from build123d import *

# Parameters (mm, degrees)
SKETCH1_R                 = 30.95625
BOSS_EXTRUDE1_DEPTH       = 50.8
CUT_EXTRUDE1_DEPTH        = 3.9624
CUT_EXTRUDE2_DEPTH        = 86.860858779
SKETCH4_R                 = 19.05
CUT_EXTRUDE3_DEPTH        = 60.630735383
SKETCH6_R                 = 23.8125
CUT_EXTRUDE4_DEPTH        = 44.45
F_4_40_TAPPED_HOLE1_D     = 2.2606
F_4_40_TAPPED_HOLE1_DEPTH = 7.62
F_4_40_TAPPED_HOLE1_TIP   = 0.679152758
SKETCH10_R                = 40.48125
BOSS_EXTRUDE3_DEPTH       = 4.7625
FILLET1_R                 = 5.08
CIRPATTERN1_COUNT         = 2
CIRPATTERN1_ANGLE         = 60
SKETCH15_R                = 3.9624
CUT_EXTRUDE5_DEPTH        = 5.08


with BuildPart() as part:
    # Sketch1 → Boss-Extrude1 (new body)
    with BuildSketch(Plane.XY):
        Circle(SKETCH1_R)
    extrude(amount=BOSS_EXTRUDE1_DEPTH)

    # Sketch2 → Cut-Extrude1 (cut)
    with BuildSketch(Plane(origin=(0, 0, 0), x_dir=(-1, 0, 0), z_dir=(0, 0, -1))):
        with BuildLine():
            Line((-18.3261, -22.2885), (18.3261, -22.2885))
            ThreePointArc((18.3261, -22.2885), (21.12793991, -21.12793991), (22.2885, -18.3261))
            Line((22.2885, -18.3261), (22.2885, 18.3261))
            ThreePointArc((22.2885, 18.3261), (21.12793991, 21.12793991), (18.3261, 22.2885))
            Line((18.3261, 22.2885), (-18.3261, 22.2885))
            ThreePointArc((-18.3261, 22.2885), (-21.12793991, 21.12793991), (-22.2885, 18.3261))
            Line((-22.2885, 18.3261), (-22.2885, -18.3261))
            ThreePointArc((-22.2885, -18.3261), (-21.12793991, -21.12793991), (-18.3261, -22.2885))
        make_face()
    extrude(amount=-CUT_EXTRUDE1_DEPTH, mode=Mode.SUBTRACT)

    # Sketch3 → Cut-Extrude2 (cut, through all)
    with BuildSketch(Plane(origin=(30.95625, 0, 0), x_dir=(0, 0, -1), z_dir=(1, 0, 0))):
        with BuildLine():
            Line((-44.45, 25.4), (0, 30.95625))
            Line((0, 30.95625), (-50.8, 30.95625))
            Line((-50.8, 30.95625), (-50.8, -30.95625))
            Line((-50.8, -30.95625), (0, -30.95625))
            Line((0, -30.95625), (-44.45, -25.4))
            ThreePointArc((-44.45, -25.4), (-19.05, 0), (-44.45, 25.4))
        make_face()
    extrude(amount=-CUT_EXTRUDE2_DEPTH, mode=Mode.SUBTRACT)

    # Sketch4 → Cut-Extrude3 (cut, through all)
    with BuildSketch(Plane(origin=(0, 0, 3.9624), x_dir=(-1, 0, 0), z_dir=(0, 0, -1))):
        Circle(SKETCH4_R)
    extrude(amount=-CUT_EXTRUDE3_DEPTH, mode=Mode.SUBTRACT)

    # Sketch6 → Cut-Extrude4 (cut)
    with BuildSketch(Plane.XY.offset(50.8)):
        Circle(SKETCH6_R)
    extrude(amount=-CUT_EXTRUDE4_DEPTH, mode=Mode.SUBTRACT)

    # #4-40 Tapped Hole1
    with Locations(Plane(origin=(0, 0, 3.9624), x_dir=(-1, 0, 0), z_dir=(0, 0, -1))):
        with Locations((-18.2626, 18.2626), (18.2626, 18.2626), (18.2626, -18.2626), (-18.2626, -18.2626)):
            Hole(F_4_40_TAPPED_HOLE1_D / 2, depth=F_4_40_TAPPED_HOLE1_DEPTH)
            with Locations((0, 0, -(F_4_40_TAPPED_HOLE1_DEPTH + F_4_40_TAPPED_HOLE1_TIP / 2))):  # 118° drill point
                Cone(0, F_4_40_TAPPED_HOLE1_D / 2, F_4_40_TAPPED_HOLE1_TIP, mode=Mode.SUBTRACT)

    # Sketch10 → Boss-Extrude3 (add)
    with BuildSketch(Plane(origin=(0, 0, 0), x_dir=(-1, 0, 0), z_dir=(0, 0, -1))):
        Circle(SKETCH10_R)
        with BuildLine():
            Line((-17.695463093, 25.4), (17.695463093, 25.4))
            ThreePointArc((17.695463093, 25.4), (30.95625, 0), (17.695463093, -25.4))
            Line((17.695463093, -25.4), (-17.695463093, -25.4))
            ThreePointArc((-17.695463093, -25.4), (-30.95625, 0), (-17.695463093, 25.4))
        make_face(mode=Mode.SUBTRACT)
    extrude(amount=-BOSS_EXTRUDE3_DEPTH)

    # Fillet1
    fillet1_edges = [part.edges().sort_by_distance(p)[0] for p in [
        (30.95625, 0, 4.7625),
        (-30.95625, 0, 4.7625),
        (0, -30.3609375, 4.7625),
        (0, 30.3609375, 4.7625),
    ]]
    fillet(fillet1_edges, radius=FILLET1_R)

    # Sketch13 → #8 Clearance Hole1 (revolve, cut)
    with BuildSketch(Plane(origin=(-18.415, 31.895715621, 4.7625), x_dir=(0, -1, 0), z_dir=(1, 0, 0))):
        Polygon((0, 0), (0, 26.750674586), (2.2479, 25.4), (2.2479, 0), align=None)
    f_8_clearance_hole1 = revolve(axis=Axis((-18.415, 31.895715621, 11.1125), (0, 0, -1)), mode=Mode.SUBTRACT)

    # CirPattern1: #8 Clearance Hole1 ×2 about axis
    cirpattern1_axis = Axis((0, 0, 4.7625), (0, 0, -1))
    for i in range(1, CIRPATTERN1_COUNT):
        add(f_8_clearance_hole1.rotate(cirpattern1_axis, i * CIRPATTERN1_ANGLE / (CIRPATTERN1_COUNT - 1)), mode=Mode.SUBTRACT)

    # Mirror1: #8 Clearance Hole1 across plane
    add(f_8_clearance_hole1.mirror(Plane.ZX), mode=Mode.SUBTRACT)

    # Mirror1 copy 1 sketch → Mirror1 copy 1 (revolve, cut)
    with BuildSketch(Plane(origin=(18.415, -31.895715621, 4.7625), x_dir=(-0.8660254037844399, 0.4999999999999978, 0), z_dir=(0.4999999999999978, 0.8660254037844399, 0))):
        Polygon((0, 0), (0, -26.750674586), (2.2479, -25.4), (2.2479, 0), align=None)
    revolve(axis=Axis((18.415, -31.895715621, 11.1125), (0, 0, 1)), mode=Mode.SUBTRACT)

    # Sketch15 → Cut-Extrude5 (cut)
    with BuildSketch(Plane.XY.offset(9.8425)):
        with Locations((-18.415, 31.895715621)):
            Circle(SKETCH15_R)
        with Locations((18.415, 31.895715621)):
            Circle(SKETCH15_R)
        with Locations((18.415, -31.895715621)):
            Circle(SKETCH15_R)
        with Locations((-18.415, -31.895715621)):
            Circle(SKETCH15_R)
    extrude(amount=-CUT_EXTRUDE5_DEPTH, mode=Mode.SUBTRACT)


solid = part.part
Geometry: final body of the model. Coordinates: model frame, mm. A direction names the side the tool comes from. Give positions to 0.01 mm unless a question says otherwise; leave off trailing zeros. Write each loop counter-clockwise with the first axis right and the second up, starting at its lowest first coordinate (ties: lowest second). Pieces come first, ordered by that corner, then holes. Notation, with made-up numbers: (86.25, 8) - (141.25, 8) arc R10 cw to (141.25, 23) - close; hole circle Ø1 at (19, 37). An arc over 180 degrees is marked (long way). Return JSON: item names as keys, results as strings. Group by question number.
1) Section A-A on x = 0. Return the cut outline in (y, z), plus the area to 3 significant figures.
2) Section D-D on z = 15.5. Return the cut outline in (x, y) (1 decimal), plus the area to 3 significant figures.
3) Section B-B on y = 0. Return the cut outline in (x, z).
4) Set-up query: faces 1 (the cylindrical face through (30.95, -0.56, 15.37)), 2 (the cylindrical face through (-17.741, -19.265, 7.826)), 3 (the cylindrical face through (-17.551, 16.094, 17.934)), 4 (the cylindrical face through (15.12, -11.59, 5.14)). Return all of +Z, -Z, +X, -X, +Y, -Y with unobstructed straight access to the full face (end or side cutting, diameter ignored); none if empty.
5) Mould query, pull axis Y, two halves, no side actions, for faces 5 (the cylindrical face through (18.784, -19.265, 7.826)), 6 (the flat face through (-26, 1, 0)), 7 (the cylindrical face through (-30.95, 0.56, 15.37)), 8 (the cylindrical face through (-13.614, -20.485, 29.432)). Classes: released by +Y, released by -Y, zero draft, split by the parting line, or undercut.
6) First-contact query: P1, Ø2.5, axis at x = 18.26, y = -18.26, coming from the -Z side; P2, Ø8, axis at x = 10.5, z = 8, coming from the +Y side; P3, Ø14.5, axis at x = -11, y = 11, coming from the +Z side; P4, Ø5, axis at x = 18.41, y = 31.9, coming from the -Z side. Flat tips, straight axial feed; report the tip coordinate or a pass-through.
7) Section C-C on z = 33.5. Return the cut outline in (x, y) (1 decimal), plus the area to 3 significant figures.
8) Line query: line 1 (Y direction, x = 3, z = 12); line 2 (Y direction, x = -17, z = 6.5); line 3 (Z direction, x = 20, y = 0). Output: solid intervals per line, ascending.
Filled in:
{
 "1": {"outline": "(-40.48, 0) - (-22.29, 0) - (-22.29, 3.96) - (-19.05, 3.96) - (-19.05, 6.35) - (-23.81, 6.35) - (-23.81, 35.61) arc R25.4 cw to (-25.4, 44.45) - (-29.8, 9.21) arc R5.08 cw to (-34.85, 4.76) - (-40.48, 4.76) - close; (19.05, 3.96) - (22.29, 3.96) - (22.29, 0) - (40.48, 0) - (40.48, 4.76) - (34.85, 4.76) arc R5.08 cw to (29.8, 9.21) - (25.4, 44.45) arc R25.4 cw to (23.81, 35.61) - (23.81, 6.35) - (19.05, 6.35) - close", "area": "506 mm^2"},
 "2": {"outline": "(-10.8, -29) - (10.8, -29) arc R31 ccw to (10.8, 29) - (-10.8, 29) arc R31 ccw to start; hole circle Ø47.6 at (0, 0)", "area": "1,170 mm^2"},
 "3": {"outline": "(-40.48, 0) - (-22.29, 0) - (-22.29, 3.96) - (-19.05, 3.96) - (-19.05, 6.35) - (-23.81, 6.35) - (-23.81, 19.05) - (-30.96, 19.05) - (-30.96, 9.84) arc R5.08 cw to (-36.04, 4.76) - (-40.48, 4.76) - close; (19.05, 3.96) - (22.29, 3.96) - (22.29, 0) - (40.48, 0) - (40.48, 4.76) - (36.04, 4.76) arc R5.08 cw to (30.96, 9.84) - (30.96, 19.05) - (23.81, 19.05) - (23.81, 6.35) - (19.05, 6.35) - close"},
 "4": {"face 1": "+Z, +X", "face 2": "-Z", "face 3": "+Z", "face 4": "+Z, -Z"},
 "5": {"face 5": "undercut", "face 6": "zero draft", "face 7": "split by the parting line", "face 8": "undercut"},
 "6": {"P1": "stops at z = 3.96", "P2": "stops at y = 39.65", "P3": "stops at z = 6.35", "P4": "stops at z = 0"},
 "7": {"outline": "(-20.8, -22.9) arc R31 ccw to (-15.5, -26.8) - (15.5, -26.8) arc R31 ccw to (20.8, -22.9) - (6.5, -22.9) arc R23.8 cw to (-6.5, -22.9) - close; (-20.8, 22.9) - (-6.5, 22.9) arc R23.8 cw to (6.5, 22.9) - (20.8, 22.9) arc R31 ccw to (15.5, 26.8) - (-15.5, 26.8) arc R31 ccw to start", "area": "267 mm^2"},
 "8": {"line 1": "y = -29.46 to -23.62, 23.62 to 29.46", "line 2": "y = -27.36 to -16.67, 16.67 to 27.36", "line 3": "z = 3.96 to 6.35"}
}
